Here's how the part is built. I have some questions about the finished solid (model axes, mm). Give positions to 0.01 mm unless a question says otherwise; leave off trailing zeros. Write each loop counter-clockwise with the first axis right and the second up, starting at its lowest first coordinate (ties: lowest second). Pieces come first, ordered by that corner, then holes. Notation, with made-up numbers: (48, 18) -> (101, 18) arc R18 ccw to (101, 43) -> close; hole circle Ø1 at (83, 87.5). An arc over 180 degrees is marked (long way). Use one line per item in the form item = value.
Autodesk Inventor part; units mm, degrees
ref_plane "YZ Plane" through (0, 0, 0) normal (1, 0, 0) x (0, 1, 0)
ref_plane "XZ Plane" through (0, 0, 0) normal (0, 1, 0) x (-1, 0, 0)
ref_plane "XY Plane" through (0, 0, 0) normal (0, 0, 1) x (1, 0, 0)
sketch "Boceto1" plane through (0, 0, 0) normal (0, 1, 0) x (-1, 0, 0)
  line L0 (51.5, 103) -> (51.5, -103)
  line L1 (-51.5, 103) -> (51.5, -103) construction
  line L2 (51.5, 103) -> (-51.5, -103) construction
  line L3 (26.5, 103) -> (26.5, 100)
  line L4 (26.5, 100) -> (-23.5, 100)
  line L5 (-23.5, 100) -> (-23.5, 103)
  line L6 (-51.5, 103) -> (-23.5, 103)
  line L7 (26.5, 103) -> (51.5, 103)
  line L8 (26.5, -103) -> (26.5, -100)
  line L9 (26.5, -100) -> (-23.5, -100)
  line L10 (-23.5, -100) -> (-23.5, -103)
  line L11 (51.5, -103) -> (26.5, -103)
  line L12 (-23.5, -103) -> (-51.5, -103)
  line L13 (-51.5, 75) -> (-48.5, 75)
  line L14 (-48.5, 75) -> (-48.5, 25)
  line L15 (-48.5, 25) -> (-51.5, 25)
  line L16 (-51.5, 75) -> (-51.5, 103)
  line L17 (-51.5, -25) -> (-48.5, -25)
  line L18 (-48.5, -25) -> (-48.5, -75)
  line L19 (-48.5, -75) -> (-51.5, -75)
  line L20 (-51.5, -103) -> (-51.5, -75)
  line L21 (-51.5, -25) -> (-51.5, 25)
  point P0 (0, 0)
  dimension "d4" = 3
  dimension "d5" = 50
  dimension "d7" = 3
  dimension "d8" = 50
  dimension "d24" = 50
  dimension "d30" = 3
  dimension "d33" = 25
  dimension "d35" = 100
  dimension "d36" = 25
  dimension "d38" = 200
extrude "Extrusión1" add sketch "Boceto1" along normal blind 3
properties part number "Piso"
Q1. I want a section at B-B, the plane x = -19. Write out the boundary of the cut face in (y, z).
Result set:
outline = (0, -100) -> (3, -100) -> (3, 100) -> (0, 100) -> close
Q2. Will this pin go through, and if not, where does the flat tip stop? pin 1 Ø0.9 at (y, z) = (2, 40.5) entering from +X.
Result set:
pin_1 = 48.5
Q3. I want a section at C-C, the plane z = 52. Write out the boundary of the cut face in (x, y).
Result set:
outline = (-51.5, 0) -> (48.5, 0) -> (48.5, 3) -> (-51.5, 3) -> close
Q4. I want a section at A-A, the plane y = 1.35. Write out the boundary of the cut face in (x, z).
Result set:
outline = (-51.5, -103) -> (-26.5, -103) -> (-26.5, -100) -> (23.5, -100) -> (23.5, -103) -> (51.5, -103) -> (51.5, -75) -> (48.5, -75) -> (48.5, -25) -> (51.5, -25) -> (51.5, 25) -> (48.5, 25) -> (48.5, 75) -> (51.5, 75) -> (51.5, 103) -> (23.5, 103) -> (23.5, 100) -> (-26.5, 100) -> (-26.5, 103) -> (-51.5, 103) -> close
Q5. If I drill on line 1 along Z through (x, y) = (-17, 0.9); line 2 along X through (y, z) = (1.1, -61), over which ranges is the centre line in solid material (lowest first)? Write a range as from..to.
Result set:
line_1 = -100..100
line_2 = -51.5..48.5
